```python
from build123d import *

# Parameters (mm, degrees)
SKETCH1_R               = 2.75
BOSS_EXTRUDE1_DEPTH     = 2
SKETCH2_R               = 1.4
BOSS_EXTRUDE2_DEPTH     = 11
SKETCH3_W               = 1
SKETCH3_H               = 1.4
CUT_EXTRUDE1_DEPTH      = 3.75
CUT_EXTRUDE1_DEPTH_BACK = 3.75


with BuildPart() as part:
    # Sketch1 → Boss-Extrude1 (new body)
    with BuildSketch(Plane(origin=(0, 0, 0), x_dir=(1, 0, 0), z_dir=(0, 1, 0))):
        Circle(SKETCH1_R)
    extrude(amount=BOSS_EXTRUDE1_DEPTH)

    # Sketch2 → Boss-Extrude2 (add)
    with BuildSketch(Plane.XZ):
        Circle(SKETCH2_R)
    extrude(amount=BOSS_EXTRUDE2_DEPTH)

    # Sketch3 → Cut-Extrude1 (cut, two sides)
    with BuildSketch(Plane(origin=(0, 0, 0), x_dir=(0, 0, -1), z_dir=(1, 0, 0))) as cut_extrude1_sk:
        with Locations((0, 1.3)):
            Rectangle(SKETCH3_W, SKETCH3_H)
    extrude(amount=CUT_EXTRUDE1_DEPTH, mode=Mode.SUBTRACT)
    extrude(cut_extrude1_sk.sketch, amount=-CUT_EXTRUDE1_DEPTH_BACK, mode=Mode.SUBTRACT)


solid = part.part
```
Build history of the part. All positions in model axes, mm. A direction names the side the tool comes from. Coordinates: 2 decimals unless noted, no trailing zeros. Order: outer loops, then holes, each group sorted by start corner. A loop starts at its lowest first (then second) coordinate and runs counter-clockwise, first axis right, second up. Notation, with made-up numbers: M 63,-39 L 96,-39 A33 ccw 96,-3 Z; hole C 23,-6 d10. An arc over 180 degrees is marked long. One line per question, with ' | ' between items. Start each with the question number.
1. Tool access for faces 1 (the face through (1.2, 0, 1.2)), 2 (the face through (0, 2, 1)), 3 (the face through (0, 1, -0.5)): list every direction of +Z, -Z, +X, -X, +Y, -Y with a clear straight run to the whole face (end or side of a thin tool).
2. Cut at B-B (x = 0). Write the cut outline in (y, z), plus the area to 3 significant figures.
3. Cut at D-D (x = -1.85). Write the cut outline in (y, z), plus the area to 3 significant figures.
4. Mould opens along Z. For faces 4 (the face through (0, 2, -1)), 5 (the face through (0, 0.6, 0)), 6 (the face through (2.62, 0.99, -0.83)) say: +Z half, -Z half, draft (parallel to the pull), parting line (faces both ways), or undercut.
5. Cut at A-A (z = 0). Write the cut outline in (x, y).
6. Flat gauge pins, fed straight in: P1, Ø3, axis at x = -0.5, y = -2.5, coming from the +Z side; P2, Ø2, axis at x = 0.5, y = -4, coming from the -Z side; P3, Ø1.5, axis at y = -1, z = 0, coming from the +X side. Where does each tip first touch, or does it go through?
7. Wall check: line 1 along Y through (x, z) = (1.2, -1.65); line 2 along Y through (x, z) = (-0.9, 0.45); line 3 along Z through (x, y) = (1.5, 1). Give the ranges that are in metal, low to high. Write a range as [from, to].
8. Cut at C-C (y = -6.5). Write the cut outline in (x, z).
The answers:
1) face 1: -Y | face 2: +Z, -Z, +X, -X, +Y | face 3: +X, -X, +Y
2) outline: M -11,-1.4 L 0,-1.4 L 0,-2.75 L 2,-2.75 L 2,-0.5 L 0.6,-0.5 L 0.6,0.5 L 2,0.5 L 2,2.75 L 0,2.75 L 0,1.4 L -11,1.4 Z | area: 40.4 mm2
3) outline: M 0,-2.03 L 2,-2.03 L 2,-0.5 L 0.6,-0.5 L 0.6,0.5 L 2,0.5 L 2,2.03 L 0,2.03 Z | area: 6.74 mm2
4) face 4: draft | face 5: undercut | face 6: parting line
5) outline: M -2.75,0 L -1.4,0 L -1.4,-11 L 1.4,-11 L 1.4,0 L 2.75,0 L 2.75,0.6 L -2.75,0.6 Z
6) P1: stops at z = 1.4 | P2: stops at z = -1.4 | P3: stops at x = 1.4
7) line 1: y = [0, 2] | line 2: y = [-11, 0.6] | line 3: z = [-2.3, -0.5], [0.5, 2.3]
8) outline: C 0,0 d2.8
